Input: part model. Units: mm. Frame: model coordinates. A direction names the side the tool comes from. Round coordinates to 2 decimals unless told otherwise and drop trailing zeros. Loops run counter-clockwise (first coordinate to the right, second up) from the corner with the lowest first, then second, coordinate; pieces in that order, holes last.
(1) First-contact query: pin 1 Ø10 at (x, y) = (-7, -15) entering from -Z; pin 2 Ø5 at (x, y) = (-8.5, -23) entering from -Z; pin 3 Ø1.5 at (y, z) = (-9.5, -3.5) entering from +X. Flat tips, straight axial feed; report the tip coordinate or a pass-through.
(2) Cut plane D-D, the plane x = 6.25. Output: boundary loops of the cut face in (y, z).
(3) Draft query along Y for faces 6 (the face through (8.8, 3, 0)), 7 (the face through (0.065, -2.465, -4.504)), 8 (the face through (-1, 2, -2)). Return one class per face: released by +Y, released by -Y, zero draft, split by the parting line, or undercut.
(4) Cut plane A-A, the plane x = 0. Output: boundary loops of the cut face in (y, z), and give its area (3 significant figures).
(5) Cut plane C-C, the plane z = -7.25. Output: boundary loops of the cut face in (x, y), and give its area (3 significant figures).
(6) Line query: line 1 (Z direction, x = 0, y = -2.85); line 2 (Z direction, x = 8.7, y = 4); line 3 (X direction, y = 1, z = -1.25). Output: solid intervals per line, ascending.
(7) Access query for faces 1 (the face through (0, 3, 0)), 2 (the face through (10.492, -12.818, 3.304)), 3 (the face through (0, -33, 0)), 4 (the face through (7.2, -0.5, -2.5)), 5 (the face through (9.9, -0.5, -2.5)). Directions: +Z, -Z, +X, -X, +Y, -Y. A direction counts if a zero-diameter tool reaches every point of the face in a straight line with its end or side. Return the directions, or none.
(8) Cut plane B-B, the plane y = -18. Output: boundary loops of the cut face in (x, z), and give its area (3 significant figures).
from build123d import *

# Parameters (mm, degrees)
F0_R      = 11
F1_DEPTH  = 26
F2_R      = 10
F3_DEPTH  = 2
F4_R      = 1
F5_DEPTH  = 5
F7_DEPTH  = 1
F9_DEPTH  = 1
F10_R     = 3
F11_DEPTH = 2
F12_R     = 2
F12_R_2   = 1
F13_DEPTH = 5
F14_DEPTH = 1
F15_R     = 0.5
F16_DEPTH = 5
F17_W     = 0.5
F17_H     = 5
F18_DEPTH = 1.5
F19_W     = 0.5
F19_H     = 3
F20_DEPTH = 5
F21_W     = 0.5
F21_H     = 5
F22_DEPTH = 1.5
F23_W     = 0.5
F23_H     = 3
F24_DEPTH = 5
F26_DEPTH = 20.001
F27_DEPTH = 20.001
F25_R     = 1
F28_DEPTH = 20.001


with BuildPart() as f1:
    # F0 (on Front) → F1 (new body)
    with BuildSketch(Plane.XZ):
        Circle(F0_R)
    extrude(amount=F1_DEPTH)

    # F2 (on face) → F3 (join)
    with BuildSketch(Plane.XZ.offset(26)):
        Circle(F2_R)
    extrude(amount=F3_DEPTH)

    # F4 (on face) → F5 (join)
    with BuildSketch(Plane.XZ.offset(28)):
        Circle(F4_R)
    extrude(amount=F5_DEPTH)

    # F6 (on face) → F7 (cut)
    with BuildSketch(Plane(origin=(0, 0, 0), x_dir=(-1, 0, 0), z_dir=(0, 1, 0))):
        with BuildLine():
            Line((-10.7121426428, -2.5), (-5.837165408, -2.5))
            ThreePointArc((-5.837165408, -2.5), (0, -6.35), (5.837165408, -2.5))
            Line((5.837165408, -2.5), (10.7121426428, -2.5))
            ThreePointArc((10.7121426428, -2.5), (10.9277987049, -1.258258902), (11, 0))
            ThreePointArc((11, 0), (10.9277987049, 1.258258902), (10.7121426428, 2.5))
            Line((10.7121426428, 2.5), (5.837165408, 2.5))
            ThreePointArc((5.837165408, 2.5), (0, 6.35), (-5.837165408, 2.5))
            Line((-5.837165408, 2.5), (-10.7121426428, 2.5))
            ThreePointArc((-10.7121426428, 2.5), (-11, 0), (-10.7121426428, -2.5))
        make_face()
    extrude(amount=-F7_DEPTH, mode=Mode.SUBTRACT)

    # F8 (on face) → F9 (join)
    with BuildSketch(Plane(origin=(0, -1, 0), x_dir=(-1, 0, 0), z_dir=(0, 1, 0))):
        with BuildLine():
            Line((-1, 6.2707655035), (-1, 3.8729833462))
            ThreePointArc((-1, 3.8729833462), (-4, 0), (-1, -3.8729833462))
            Line((-1, -3.8729833462), (-1, -6.2707655035))
            ThreePointArc((-1, -6.2707655035), (0, -6.35), (1, -6.2707655035))
            Line((1, -6.2707655035), (1, -3.8729833462))
            ThreePointArc((1, -3.8729833462), (4, 0), (1, 3.8729833462))
            Line((1, 3.8729833462), (1, 6.2707655035))
            ThreePointArc((1, 6.2707655035), (0, 6.35), (-1, 6.2707655035))
        make_face()
    extrude(amount=F9_DEPTH)

    # F10 (on face) → F11 (join)
    with BuildSketch(Plane(origin=(0, 0, 0), x_dir=(-1, 0, 0), z_dir=(0, 1, 0))):
        Circle(F10_R)
    extrude(amount=F11_DEPTH)

    # F12 (on face) → F13 (cut)
    with BuildSketch(Plane(origin=(0, 2, 0), x_dir=(-1, 0, 0), z_dir=(0, 1, 0))):
        Circle(F12_R)
        Circle(F12_R_2, mode=Mode.SUBTRACT)
    extrude(amount=-F13_DEPTH, mode=Mode.SUBTRACT)

    # F14 (add): a face of the model
    f14_faces = [f1.faces().sort_by_distance(p)[0] for p in [
        (0, 2, 0),
    ]]
    extrude(f14_faces, amount=F14_DEPTH)

    # F15 (on face) → F16 (cut)
    with BuildSketch(Plane(origin=(0, 0, 0), x_dir=(-1, 0, 0), z_dir=(0, 1, 0))):
        with Locations((0, -5)):
            Circle(F15_R)
    extrude(amount=-F16_DEPTH, mode=Mode.SUBTRACT)

    # F17 (on face) → F18 (join)
    with BuildSketch(Plane(origin=(0, -1, 0), x_dir=(-1, 0, 0), z_dir=(0, 1, 0))):
        with Locations((-8.75, 0)):
            Rectangle(F17_W, F17_H)
    extrude(amount=F18_DEPTH)

    # F19 (on face) → F20 (join)
    with BuildSketch(Plane(origin=(0, 0.5, 0), x_dir=(-1, 0, 0), z_dir=(0, 1, 0))):
        with Locations((-8.75, 0)):
            Rectangle(F19_W, F19_H)
    extrude(amount=F20_DEPTH)

    # F21 (on face) → F22 (join)
    with BuildSketch(Plane(origin=(0, -1, 0), x_dir=(-1, 0, 0), z_dir=(0, 1, 0))):
        with Locations((9, 0)):
            Rectangle(F21_W, F21_H)
    extrude(amount=F22_DEPTH)

    # F23 (on face) → F24 (join)
    with BuildSketch(Plane(origin=(0, 0.5, 0), x_dir=(-1, 0, 0), z_dir=(0, 1, 0))):
        with Locations((9, 0)):
            Rectangle(F23_W, F23_H)
    extrude(amount=F24_DEPTH)

    # F25 (on face) → F26 (cut, through all)
    with BuildSketch(Plane.YZ.offset(9)):
        with BuildLine():
            ThreePointArc((4, 1.5), (5.0606601718, 1.0606601718), (5.5, 0))
            Line((5.5, 0), (5.5, 1.5))
            Line((5.5, 1.5), (4, 1.5))
        make_face()
    extrude(amount=-F26_DEPTH, mode=Mode.SUBTRACT)

    # F25 (on face) → F27 (cut, through all)
    with BuildSketch(Plane.YZ.offset(9)):
        with BuildLine():
            ThreePointArc((5.5, 0), (5.0606601718, -1.0606601718), (4, -1.5))
            Line((4, -1.5), (5.5, -1.5))
            Line((5.5, -1.5), (5.5, 0))
        make_face()
    extrude(amount=-F27_DEPTH, mode=Mode.SUBTRACT)

    # F25 (on face) → F28 (cut, through all)
    with BuildSketch(Plane.YZ.offset(9)):
        with Locations((4, 0)):
            Circle(F25_R)
    extrude(amount=-F28_DEPTH, mode=Mode.SUBTRACT)


solid = f1.part
Reported:
1. pin 1: stops at z = -10.82
1. pin 2: stops at z = -9.22
1. pin 3: stops at x = 10.65
2. outline: (-28, -7.81) - (-26, -7.81) - (-26, -9.05) - (0, -9.05) - (0, -2.5) - (-1, -2.5) - (-1, 2.5) - (0, 2.5) - (0, 9.05) - (-26, 9.05) - (-26, 7.81) - (-28, 7.81) - close
3. face 6: undercut
3. face 7: zero draft
3. face 8: released by +Y
4. outline: (-33, -1) - (-28, -1) - (-28, -10) - (-26, -10) - (-26, -11) - (0, -11) - (0, -5.5) - (-5, -5.5) - (-5, -4.5) - (0, -4.5) - (0, -3) - (2, -3) - (2, -2) - (-3, -2) - (-3, -1) - (3, -1) - (3, 1) - (-3, 1) - (-3, 2) - (2, 2) - (2, 3) - (0, 3) - (0, 11) - (-26, 11) - (-26, 10) - (-28, 10) - (-28, 1) - (-33, 1) - close
4. area: 621 mm2
5. outline: (-8.27, -26) - (-6.89, -26) - (-6.89, -28) - (6.89, -28) - (6.89, -26) - (8.27, -26) - (8.27, 0) - (-8.27, 0) - close
5. area: 458 mm2
6. line 1: z = -11 to -5.5, -4.5 to -2, -1 to 1, 2 to 11
6. line 2: z = -1.5 to -1, 1 to 1.5
6. line 3: x = -9.25 to -8.75, -2.73 to -1.56, 1.56 to 2.73, 8.5 to 9
7. face 1: +Z, -Z, +Y
7. face 2: +Y, -Y
7. face 3: +Z, -Z, +X, -X, -Y
7. face 4: +Y
7. face 5: +X, +Y
8. outline: circle Ø22 at (0, 0)
8. area: 380 mm2
